```python
from build123d import *

# Parameters (mm, degrees)
F0_W        = 21
F0_H        = 135
F1_DEPTH    = 4
F3_DEPTH    = 4.001
F4_T1_DEPTH = 159.4948974279


# Not quite as in the source:
# - a fillet or chamfer that OpenCascade refuses, or shapes differently, is made with other operations: its cross-section is extruded or revolved along the edge and cut away or added


with BuildPart() as f1:
    # F0 (on Top) → F1 (new body)
    with BuildSketch(Plane.XY):
        Rectangle(F0_W, F0_H)
    extrude(amount=F1_DEPTH)

    # F2 (on face) → F3 (cut, through all)
    with BuildSketch(Plane.XY.offset(4)):
        Polygon((10.5, 67.5), (-10.5, 67.5), (10.5, 46.5), align=None)
        Polygon((10.5, -46.5), (-10.5, -67.5), (10.5, -67.5), align=None)
    extrude(amount=-F3_DEPTH, mode=Mode.SUBTRACT)

    # F4: fillet of radius 5 on 1 edges, made by hand

    # F4_s2 → F4_t1 (cut)
    with BuildSketch(Plane.XZ.offset(-79.7474487139)):
        with BuildLine():
            ThreePointArc((-5.6010205144, 4), (-8.7632981746, 2.8729833462), (-10.5, 0))
            Line((-10.5, 0), (-10.5, 4))
            Line((-10.5, 4), (-5.6010205144, 4))
        make_face()
    extrude(amount=F4_T1_DEPTH, mode=Mode.SUBTRACT)


solid = f1.part
```
Part model, mm, in its own coordinate system. Round coordinates to 2 decimals unless told otherwise and drop trailing zeros. Write each loop counter-clockwise with the first axis right and the second up, starting at its lowest first coordinate (ties: lowest second). Pieces come first, ordered by that corner, then holes. Notation, with made-up numbers: M 76,-33.5 L 116,-33.5 A25 ccw 116,-0.5 Z; hole C 42.25,-19 d7. An arc over 180 degrees is marked long. Answer as CSV lines item,"result". Start each with the question number.
1) Drill centre lines: L1, parallel to X at y = 30, z = 3.4; L2, parallel to X at y = -11, z = 1.15; L3, parallel to Z at x = -8, y = 17.5. Where is each one in solid material? Low to high.
2) Band-saw the part on B-B (y = 5.5). List the corners of the cut face in (x, z), then the cut area to 3 significant figures.
3) Band-saw the part on A-A (x = -1.5). List the corners of the cut face in (y, z), then the cut area to 3 significant figures.
4) Drop a flat-ended pin along its axis: pin 1 (2 mm diameter, centred on x = -8, z = 1, fed in from +Y). Give the stop position or say it passes through.
Worked out:
1,L1,"-7.98 to 10.5"
1,L2,"-10.12 to 10.5"
1,L3,"0 to 3.39"
2,outline,"M -10.5,0 L 10.5,0 L 10.5,4 L -5.6,4 A5 ccw Z"
2,area,"79.1 mm²"
3,outline,"M -58.5,0 L 58.5,0 L 58.5,4 L -58.5,4 Z"
3,area,"468 mm²"
4,pin 1,"y = 66"
